```python
from build123d import *

# Parameters (mm, degrees)
F0_W     = 36
F0_H     = 20
F1_DEPTH = 4
F3_DEPTH = 20
F5_DEPTH = 15


with BuildPart() as f1:
    # F0 (on Top) → F1 (new body)
    with BuildSketch(Plane.XY):
        with Locations((18, 10)):
            Rectangle(F0_W, F0_H)
    extrude(amount=F1_DEPTH)

    # F2 (on face) → F3 (join)
    with BuildSketch(Plane.XY.offset(4)):
        Polygon((36, 20), (0, 20), (0, 18), (34, 18), (34, 0), (36, 0), align=None)
    extrude(amount=F3_DEPTH)

    # F4 (on face) → F5 (join)
    with BuildSketch(Plane.XY.offset(4)):
        with BuildLine():
            ThreePointArc((19.20947, 10.169719), (17, 11.5), (14.79053, 10.169719))
            Line((14.79053, 10.169719), (17, 9))
            Line((17, 9), (19.20947, 10.169719))
        make_face()
        with BuildLine():
            Line((17, 9), (14.79053, 10.169719))
            ThreePointArc((14.79053, 10.169719), (14.5, 9), (14.79053, 7.830281))
            Line((14.79053, 7.830281), (17, 9))
        make_face()
        with BuildLine():
            Line((19.20947, 10.169719), (17, 9))
            Line((17, 9), (19.20947, 7.830281))
            ThreePointArc((19.20947, 7.830281), (19.426281, 8.39737), (19.5, 9))
            ThreePointArc((19.5, 9), (19.426281, 9.60263), (19.20947, 10.169719))
        make_face()
        with BuildLine():
            Line((19.20947, 7.830281), (17, 9))
            Line((17, 9), (14.79053, 7.830281))
            ThreePointArc((14.79053, 7.830281), (17, 6.5), (19.20947, 7.830281))
        make_face()
    extrude(amount=F5_DEPTH)


solid = f1.part
```
Part model, mm, in its own coordinate system. A direction names the side the tool comes from. Give positions to 0.01 mm unless a question says otherwise; leave off trailing zeros. Order: outer loops, then holes, each group sorted by start corner. A loop starts at its lowest first (then second) coordinate and runs counter-clockwise, first axis right, second up. Notation, with made-up numbers: (41.25, -34) - (97.25, -34) arc R4 cw to (97.25, -28) - close; hole circle Ø4 at (-23, 10). An arc over 180 degrees is marked (long way). Use one line per item in the form item = value.
Item 1: Slice it at C-C on y = 2.75. Give the cut face in (x, z).
Solution:
outline = (0, 0) - (36, 0) - (36, 24) - (34, 24) - (34, 4) - (0, 4) - close
Item 2: Pin check, flat tips, straight feed: pin 1 Ø4 at (x, y) = (30, 17) entering from -Z; pin 2 Ø6 at (x, y) = (9, 14.5) entering from +Z; pin 3 Ø6 at (x, z) = (21.5, 14.5) entering from -Y; pin 4 Ø1.5 at (x, y) = (18, 8) entering from +Z. Stop position of each tip, or through.
Solution:
pin_1 = 0
pin_2 = 4
pin_3 = 7
pin_4 = 19
Item 3: Slice it at A-A on z = 13. Give the cut face in (x, y).
Solution:
outline = (0, 18) - (34, 18) - (34, 0) - (36, 0) - (36, 20) - (0, 20) - close; (19.21, 7.83) arc R2.5 ccw to (19.5, 9) arc R2.5 ccw to (19.21, 10.17) arc R2.5 ccw (long way) to start
Item 4: Slice it at D-D on z = 22.5. Give the cut face in (x, y), and give its area (3 significant figures).
Solution:
outline = (0, 18) - (34, 18) - (34, 0) - (36, 0) - (36, 20) - (0, 20) - close
area = 108 mm2
Item 5: Which spindle directions (+Z, -Z, +X, -X, +Y, -Y) get a long thin tool onto all of the face, cutting with end or side? Do faces 4 (the face through (34, 9, 14)), 5 (the face through (18, 20, 12)), 6 (the face through (17, 9, 19)). Say none if no direction does.
Solution:
face_4 = +Z, -Y
face_5 = +Z, -Z, +X, -X, +Y
face_6 = +Z, -X, -Y
Item 6: Two-plate mould, pull along X, no slides. Class faces 1 (the face through (36, 10, 12)), 2 (the face through (19, 0, 3)), 3 (the face through (13, 9, 4)): released by +X, released by -X, zero draft, split by the parting line, or undercut.
Solution:
face_1 = released by +X
face_2 = zero draft
face_3 = undercut
Item 7: Probe probe 1 along X at (y, z) = (3.5, 15); probe 2 along Z at (x, y) = (7, 12.75); probe 3 along Y at (x, z) = (13.5, 18). List the from-to ranges inside material, lowest first. Write a range as from..to.
Solution:
probe_1 = 34..36
probe_2 = 0..4
probe_3 = 18..20
Item 8: Slice it at B-B on x = 17.5. Give the cut face in (y, z).
Solution:
outline = (0, 0) - (20, 0) - (20, 24) - (18, 24) - (18, 4) - (11.45, 4) - (11.45, 19) - (6.55, 19) - (6.55, 4) - (0, 4) - close
